Autodesk Inventor part; units mm, degrees
ref_plane "YZ Plane" through (0, 0, 0) normal (1, 0, 0) x (0, 1, 0)
ref_plane "XZ Plane" through (0, 0, 0) normal (0, 1, 0) x (-1, 0, 0)
ref_plane "XY Plane" through (0, 0, 0) normal (0, 0, 1) x (1, 0, 0)
sketch "Sketch1" plane through (0, 0, 0) normal (0, 1, 0) x (-1, 0, 0)
  circle A0 centre (0, 0) radius 93.4
  circle A1 centre (0, 0) radius 90.4
  circle A2 centre (0, 0) radius 96.4
  dimension "d0" = 186.8
  dimension "d1" = 3
  dimension "d2" = 3
extrude "Extrusion1" add sketch "Sketch1" along normal blind 11 contours A0
extrude "Extrusion2" add sketch "Sketch1" along normal blind 3 contours A2
sketch "Sketch2" plane through (0, 3, 0) normal (0, 1, 0) x (1, 0, 0)
  circle A0 centre (-4.5, -94.2927) radius 1
  circle A1 centre (0, 0) radius 93.4
  circle A2 centre (0, 0) radius 95.4 construction
  circle A3 centre (4.5, -96.2949) radius 1
  dimension "d7" = 2
  dimension "d8" = 4.5
  dimension "d9" = 4.5
extrude "Extrusion3" cut sketch "Sketch2" against normal up to surface (3 mm away) contours A0 | A3
extrude "Extrusion4" add sketch "Sketch1" along normal blind 3 contours A1
sketch "Sketch3" plane through (0, 0, 0) normal (0, -1, 0) x (1, 0, 0)
  line L0 (96.4, -7.5) -> (76.4, -7.5)
  line L1 (76.4, -7.5) -> (76.4, 7.5)
  line L2 (76.4, 7.5) -> (96.4, 7.5)
  line L3 (96.4, 7.5) -> (96.4, -7.5)
  arc A0 (3.5009, 96.3364) -> (5.4987, 96.2431) centre (0, 0) ccw
  point P0 (96.4, 0)
  dimension "d14" = 15
  dimension "d15" = 20
extrude "Extrusion5" cut sketch "Sketch3" against normal up to surface (11 mm away) contours L0 A0 L3 | L0 L1 L2 A0 L3 | A0 L2 L3
pattern_circular "Circular Pattern1" count 3 over 180 about axis through (0, -10, 0) along (0, 1, 0) of "Extrusion5"
fillet "Fillet1" radius 3 6 edges at (76.4, 1.5, 7.5) (76.4, 1.5, -7.5) (-76.4, 1.5, 7.5) (-76.4, 1.5, -7.5) (7.5, 1.5, -76.4) (-7.5, 1.5, -76.4)
properties part number "122mm-CoilForm_3DPrint"
Source: CAD feature listing. Evaluate the final solid. Frame: model axes, mm. A direction names the side the tool comes from. Give positions to 0.01 mm unless a question says otherwise; leave off trailing zeros. Order: outer loops, then holes, each group sorted by start corner. A loop starts at its lowest first (then second) coordinate and runs counter-clockwise, first axis right, second up.
(1) Section query D-D (x = 23.5). Return the cut outline in (y, z), plus the area to 3 significant figures.
(2) Section query C-C (z = -54). Return the cut outline in (x, y), plus the area to 3 significant figures.
(3) Section query A-A (y = 6.25). Return the cut outline in (x, z).
(4) Section query B-B (x = -82). Return the cut outline in (y, z).
(5) Pull-direction query (Z, two-part tool) for faces 1 (the face through (-88, 2, 7.5)), 2 (the face through (68.14, 1.48, 68.19)), 3 (the face through (65, 3, -68)); classes: +Z half, -Z half, draft (parallel to the pull), parting line (faces both ways), or undercut.
(6) Material intervals for line 1 along Z through (x, y) = (-4.5, 2.05); line 2 along Y through (x, z) = (11, 44); line 3 along X through (y, z) = (3.25, -44.5), sorted ascending.
(7) Contact query for flat-ended pins moving along their axis: P1, Ø2, axis at x = -31, z = -4.5, coming from the +Y side; P2, Ø1, axis at x = 30.5, y = 1.5, coming from the -Z side; P3, Ø3, axis at x = -46, y = 8, coming from the -Z side; P4, Ø2, axis at x = -58.5, z = 53, coming from the -Y side. Output: stop coordinate, or through.
(8) Access query for faces 4 (the face through (-88, 2, -7.5)), 5 (the face through (-65, 3, -68)), 6 (the face through (-7.5, 2, -88)), 7 (the face through (1.95, 6.94, 93.38)), 8 (the face through (-64.55, 6.94, -63.29)). Directions: +Z, -Z, +X, -X, +Y, -Y. A direction counts if a zero-diameter tool reaches every point of the face in a straight line with its end or side. Return the directions, or none.
Outcome:
1. outline: (0, -93.49) - (3, -93.49) - (3, -90.4) - (11, -90.4) - (11, -87.29) - (3, -87.29) - (3, 87.29) - (11, 87.29) - (11, 90.4) - (3, 90.4) - (3, 93.49) - (0, 93.49) - close
1. area: 611 mm2
2. outline: (-79.86, 0) - (79.86, 0) - (79.86, 3) - (76.21, 3) - (76.21, 11) - (72.5, 11) - (72.5, 3) - (-72.5, 3) - (-72.5, 11) - (-76.21, 11) - (-76.21, 3) - (-79.86, 3) - close
2. area: 538 mm2
3. outline: (-93.1, -7.5) arc R93.4 ccw to (-7.5, -93.1) - (-7.5, -90.09) arc R90.4 cw to (-90.09, -7.5) - close; (-93.1, 7.5) - (-90.09, 7.5) arc R90.4 cw to (90.09, 7.5) - (93.1, 7.5) arc R93.4 ccw to start; (7.5, -93.1) arc R93.4 ccw to (93.1, -7.5) - (90.09, -7.5) arc R90.4 cw to (7.5, -90.09) - close
4. outline: (0, -50.68) - (3, -50.68) - (3, -44.72) - (11, -44.72) - (11, -38.05) - (3, -38.05) - (3, -7.5) - (0, -7.5) - close; (0, 7.5) - (3, 7.5) - (3, 38.05) - (11, 38.05) - (11, 44.72) - (3, 44.72) - (3, 50.68) - (0, 50.68) - close
5. face 1: undercut
5. face 2: +Z half
5. face 3: draft
6. line 1: z = -76.4 to 93.29, 95.29 to 96.29
6. line 2: y = 0 to 3
6. line 3: x = -82.12 to -78.69, 78.69 to 82.12
7. P1: stops at y = 3
7. P2: stops at z = -91.61
7. P3: stops at z = -82.12
7. P4: stops at y = 0
8. face 4: -X, +Y, -Y
8. face 5: -Z, -X, +Y
8. face 6: -Z, +Y, -Y
8. face 7: +Z, +Y
8. face 8: +Y
